from build123d import *

# Parameters (mm, degrees)
SKETCH1_W           = 714
SKETCH1_H           = 400
BOSS_EXTRUDE1_DEPTH = 18
SKETCH2_W           = 9
SKETCH2_H           = 400
CUT_EXTRUDE1_DEPTH  = 9
SKETCH3_W           = 19
SKETCH3_H           = 400
CUT_EXTRUDE2_DEPTH  = 9


with BuildPart() as part:
    # Sketch1 → Boss-Extrude1 (new body)
    with BuildSketch(Plane(origin=(0, 0, 0), x_dir=(1, 0, 0), z_dir=(0, 1, 0))):
        Rectangle(SKETCH1_W, SKETCH1_H)
    extrude(amount=BOSS_EXTRUDE1_DEPTH)

    # Sketch2 → Cut-Extrude1 (cut)
    with BuildSketch(Plane(origin=(0, 18, 0), x_dir=(1, 0, 0), z_dir=(0, 1, 0))):
        with Locations((352.5, 0)):
            Rectangle(SKETCH2_W, SKETCH2_H)
        with Locations((-352.5, 0)):
            Rectangle(SKETCH2_W, SKETCH2_H)
    extrude(amount=-CUT_EXTRUDE1_DEPTH, mode=Mode.SUBTRACT)

    # Sketch3 → Cut-Extrude2 (cut)
    with BuildSketch(Plane(origin=(0, 18, 0), x_dir=(1, 0, 0), z_dir=(0, 1, 0))):
        Rectangle(SKETCH3_W, SKETCH3_H)
    extrude(amount=-CUT_EXTRUDE2_DEPTH, mode=Mode.SUBTRACT)


solid = part.part
The model under review builds one solid part; all positions refer to its coordinate system, in mm. Give positions to 0.01 mm unless a question says otherwise; leave off trailing zeros. Write each loop counter-clockwise with the first axis right and the second up, starting at its lowest first coordinate (ties: lowest second). Pieces come first, ordered by that corner, then holes.
1. Add section A-A, the plane y = 12.75. Write out the cut boundary in (x, z), plus the area to 3 significant figures.
2. Add section B-B, the plane z = -5. Write out the cut boundary in (x, y).
3. For P1, Ø3, axis at y = 11, z = 72.5, coming from the +X side; P2, Ø7, axis at x = -353, z = 17, coming from the +Y side; P3, Ø7, axis at y = 13.5, z = 28.5, coming from the -X side, all flat-tipped, find the tip position at first contact; note any pin that passes through.
4. Wall thickness on L1, parallel to X at y = 12.5, z = 114.5: over which ranges is the line inside the solid? List them lowest first.
5. Draft analysis for pull direction X (two halves, no side actions). For faces 1 (the flat face through (0, 9, -3)), 2 (the flat face through (-5, 7, -200)), state which applies: +X half, -X half, draft (parallel to the pull), parting line (faces both ways), or undercut.
Worked answers:
1. outline: (-348, -200) - (-9.5, -200) - (-9.5, 200) - (-348, 200) - close; (9.5, -200) - (348, -200) - (348, 200) - (9.5, 200) - close
1. area: 271,000 mm2
2. outline: (-357, 0) - (357, 0) - (357, 9) - (348, 9) - (348, 18) - (9.5, 18) - (9.5, 9) - (-9.5, 9) - (-9.5, 18) - (-348, 18) - (-348, 9) - (-357, 9) - close
3. P1: stops at x = 348
3. P2: stops at y = 9
3. P3: stops at x = -348
4. L1: x = -348 to -9.5, 9.5 to 348
5. face 1: undercut
5. face 2: draft
